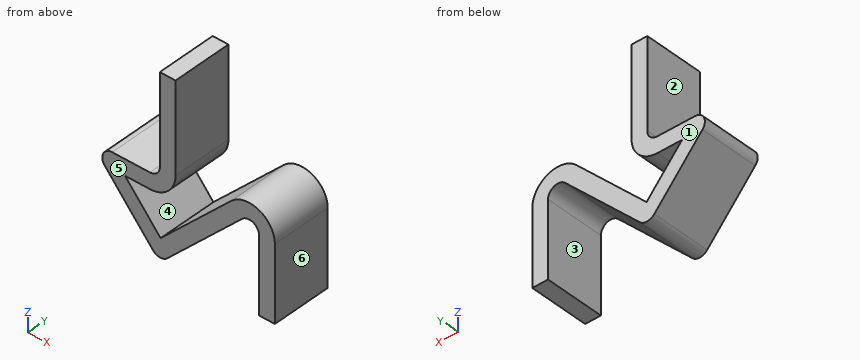
```python
from build123d import *

# Parameters (mm, degrees)
BOSS_EXTRUDE2_DEPTH = 1.5


with BuildPart() as part:
    # Sketch8 → Boss-Extrude2 (new, symmetric)
    with BuildSketch(Plane(origin=(0, 0, 0), x_dir=(1, 0, 0), z_dir=(0, 1, 0))):
        with BuildLine():
            Line((0, 0), (0, 4.5))
            ThreePointArc((0, 4.5), (-0.146446609, 4.853553391), (-0.5, 5))
            Line((-0.5, 5), (-2.398115887, 5))
            ThreePointArc((-2.398115887, 5), (-2.853432344, 5.293391859), (-2.774404234, 5.829252304))
            Line((-2.774404234, 5.829252304), (-0.351933318, 8.597790494))
            ThreePointArc((-0.351933318, 8.597790494), (0.007716061, 8.768261258), (0.37790842, 8.62209158))
            Line((0.37790842, 8.62209158), (4.146446609, 4.853553391))
            ThreePointArc((4.146446609, 4.853553391), (4.691341716, 4.745167015), (5, 5.207106781))
            Line((5, 5.207106781), (5, 9))
            Line((5, 9), (5.79375, 9))
            Line((5.79375, 9), (5.79375, 5.207106781))
            ThreePointArc((5.79375, 5.207106781), (4.995096691, 4.011837636), (3.585180602, 4.292287383))
            Line((3.585180602, 4.292287383), (0.038663609, 7.838804376))
            Line((0.038663609, 7.838804376), (-1.75075897, 5.79375))
            Line((-1.75075897, 5.79375), (-0.5, 5.79375))
            ThreePointArc((-0.5, 5.79375), (0.414819398, 5.414819398), (0.79375, 4.5))
            Line((0.79375, 4.5), (0.79375, 0))
            Line((0.79375, 0), (0, 0))
        make_face()
    extrude(amount=BOSS_EXTRUDE2_DEPTH, both=True)


solid = part.part
```
CAD build for the part. Positions are in the model's coordinates, mm. Face numbers are marked on the shaded views. A direction names the side the tool comes from. Coordinates: 2 decimals unless noted, no trailing zeros. Order: outer loops, then holes, each group sorted by start corner. A loop starts at its lowest first (then second) coordinate and runs counter-clockwise, first axis right, second up.
(1) Pin check, flat tips, straight feed: pin 1 Ø1.5 at (x, y) = (-1.5, 0) entering from +Z; pin 2 Ø1.5 at (y, z) = (0.5, -7.5) entering from -X; pin 3 Ø1.4 at (x, y) = (-1, -0.5) entering from -Z. Stop position of each tip, or through.
Solution:
pin 1: stops at z = -5
pin 2: stops at x = -1.97
pin 3: stops at z = -8.65
(2) Saw through at B-B, the plane x = 0.25. Write the cut outline in (y, z).
Solution:
outline: (-1.5, -8.71) - (1.5, -8.71) - (1.5, -7.63) - (-1.5, -7.63) - close; (-1.5, -5.55) - (1.5, -5.55) - (1.5, 0) - (-1.5, 0) - close
(3) Mould opens along X. For the marked faces 4, 5 and 6 say: released by +X, released by -X, zero draft, split by the parting line, or undercut.
Solution:
face 4: undercut
face 5: zero draft
face 6: released by +X
(4) Saw through at A-A, the plane z = -7.25. Write the cut outline in (x, y).
Solution:
outline: (-1.53, -1.5) - (-0.48, -1.5) - (-0.48, 1.5) - (-1.53, 1.5) - close; (0.63, -1.5) - (1.75, -1.5) - (1.75, 1.5) - (0.63, 1.5) - close; (5, -1.5) - (5.79, -1.5) - (5.79, 1.5) - (5, 1.5) - close
(5) Which spindle directions (+Z, -Z, +X, -X, +Y, -Y) get a long thin tool onto all of the face, cutting with end or side? Do the marked faces 1, 2 and 3. Say none if no direction does.
Solution:
face 1: +Z, -Z, +X, -X, +Y
face 2: +Z, -X, +Y, -Y
face 3: -Z, +Y, -Y
(6) Saw through at C-C, the plane y = 0.5. Write the cut outline in (x, z), and give its area (3 significant figures).
Solution:
outline: (-2.77, -5.83) - (-0.35, -8.6) arc R0.5 ccw to (0.38, -8.62) - (4.15, -4.85) arc R0.5 cw to (5, -5.21) - (5, -9) - (5.79, -9) - (5.79, -5.21) arc R1.29 ccw to (3.59, -4.29) - (0.04, -7.84) - (-1.75, -5.79) - (-0.5, -5.79) arc R1.29 ccw to (0.79, -4.5) - (0.79, 0) - (0, 0) - (0, -4.5) arc R0.5 cw to (-0.5, -5) - (-2.4, -5) arc R0.5 ccw to start
area: 18.2 mm2
(7) Saw through at D-D, the plane x = -0.75. Write the cut outline in (y, z), and give its area (3 significant figures).
Solution:
outline: (-1.5, -8.14) - (1.5, -8.14) - (1.5, -6.94) - (-1.5, -6.94) - close; (-1.5, -5.79) - (1.5, -5.79) - (1.5, -5) - (-1.5, -5) - close
area: 6.00 mm2
(8) Drill centre lines: L1, parallel to X at y = -0.2, z = -7.5; L2, parallel to X at y = 1.35, z = -5.25; L3, parallel to Z at x = 4.5, y = 1.25. Where is each one in solid material? Low to high.
Solution:
L1: x = -1.31 to -0.26, 0.38 to 1.5, 5 to 5.79
L2: x = -2.83 to 0.55, 2.63 to 3.75, 5 to 5.79
L3: z = -4.71 to -3.91
